from build123d import *

# Parameters (mm, degrees)
F3_R = 5.08


# Not quite as in the source:
# - a variable given as a bare number and used for a length is read in inches; the dataset says mm whatever the document's units were


with BuildPart() as f2:
    # F1 (on Front) → F2 (revolve)
    with BuildSketch(Plane.XZ):
        Polygon((-25.4, 46.355), (0, 31.6153030303), (50.8, 32.385), (50.8, 36.195), (0, 36.195), (-25.4, 50.38725), (-28.575, 53.56225), (-31.75, 50.38725), (-76.2, 50.165), (-76.2, 46.355), align=None)
    revolve(axis=Axis((-24.3991323134, 0, 0), (-1, 0, 0)))

    # F3
    f3_edges = [f2.edges().sort_by_distance(p)[0] for p in [
        (-25.4, 0, -46.355),
        (0, 0, -31.615303),
        (0, 0, -36.195),
        (-31.75, 0, -50.38725),
        (-25.4, 0, -50.38725),
    ]]
    fillet(f3_edges, radius=F3_R)


solid = f2.part
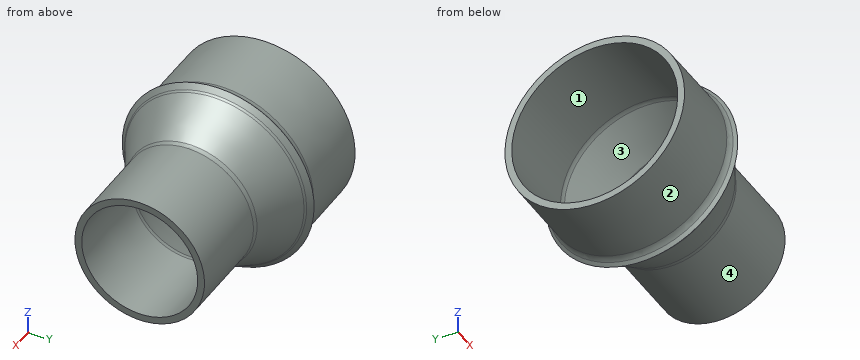
Check sheet for the modelled part. Datum: model origin and axes. Units: mm. Face numbers are marked on the shaded views. A direction names the side the tool comes from. Coordinates: 2 decimals unless noted, no trailing zeros. Loops run counter-clockwise (first coordinate to the right, second up) from the corner with the lowest first, then second, coordinate; pieces in that order, holes last. Notation, with made-up numbers: (6, -5) -> (16, -5) arc R30 cw to (16, 29) -> close; hole circle Ø10 at (68, 66.25). An arc over 180 degrees is marked (long way). Answer in a Markdown table with one row per item.
1. Sectioned sample at A-A, the plane x = -14. Record the boundary of the cut face in (y, z) (1 decimal), then the cut area to 3 significant figures.
Check values:
| item | result |
|---|---|
| outline | circle Ø88 at (0, 0); hole circle Ø79.5 at (0, 0) |
| area | 1,130 mm2 |
2. Material ranges on line 1 along Y through (x, z) = (-37.5, 0) (1 decimal); line 2 along Z through (x, y) = (-63, 0) (3 decimals); line 3 along Z through (x, y) = (-54, 0) (3 decimals), recorded low to high. Write a range as [from, to].
Check values:
| item | result |
|---|---|
| line 1 | y = [-50.4, -46.4], [46.4, 50.4] |
| line 2 | z = [-50.231, -46.355], [46.355, 50.231] |
| line 3 | z = [-50.276, -46.355], [46.355, 50.276] |
3. Release check for a two-part mould opening along Y. For the marked faces 1 and 2 record: released by +Y, released by -Y, zero draft, split by the parting line, or undercut.
Check values:
| item | result |
|---|---|
| face 1 | undercut |
| face 2 | split by the parting line |
4. Go/stop test with flat-tipped pins: pin 1 (3 mm diameter, centred on x = -22.5, z = 26, fed in from -Y); pin 2 (1 mm diameter, centred on y = 36, z = 35, fed in from +X); pin 3 (6 mm diameter, centred on x = -8, z = 24.5, fed in from +Y). Record where each tip stops, or that it passes through.
Check values:
| item | result |
|---|---|
| pin 1 | stops at y = -42.6 |
| pin 2 | stops at x = -24.19 |
| pin 3 | stops at y = 35.37 |
5. Access from +Z, -Z, +X, -X, +Y, -Y to the whole of each face (thin tool, end or side, straight path). Record for the marked faces 3 and 4.
Check values:
| item | result |
|---|---|
| face 3 | -X |
| face 4 | +X |
